The model under review builds one solid part; all positions refer to its coordinate system, in mm. Round coordinates to 2 decimals unless told otherwise and drop trailing zeros. Order: outer loops, then holes, each group sorted by start corner. A loop starts at its lowest first (then second) coordinate and runs counter-clockwise, first axis right, second up. Notation, with made-up numbers: M 27.25,27.25 L 83.25,27.25 A33 cw 83.25,61.25 Z; hole C -8.5,6.5 d8. An arc over 180 degrees is marked long. Answer as a JSON object with one key per item and string values. Group by question number.
1) Consider section A-A, the plane y = 1.5. Count the separate pieces of the cut face and the enclosed holes in it, then the cut area to 3 significant figures.
2) The part is to be moulded in two halves that separate along X. For faces 1 (the flat face through (69.85, 13, 11)), 2 (the flat face through (5, 3.175, -2)), 3 (the flat face through (-47.5, 1.6, -3.3)), 4 (the cylindrical face through (27.93, 1.57, -0.33)), say which applies: +X half, -X half, draft (parallel to the pull), parting line (faces both ways), or undercut.
3) Insertion check: pin 1 Ø8 at (x, z) = (-25.4, 0) entering from +Y (3 decimals); pin 2 Ø6 at (x, y) = (44.45, 17.46) entering from -Z (3 decimals); pin 3 Ø8 at (y, z) = (5.5, -2.5) entering from +X. Each pin has a flat end and moves straight along its axis. Give the tip position at first contact, or say it passes through.
4) Consider section D-D, the plane x = 19.05. Write out the cut boundary in (y, z) (3 decimals).
5) Consider section C-C, the plane z = 4.5. Write out the cut boundary in (x, y) (3 decimals), then the cut area to 3 significant figures.
6) To check wall thickness, follow line 1 (Y direction, x = -44.45, z = 10.7); line 2 (Y direction, x = 16.5, z = 0.5) (3 decimals); line 3 (Z direction, x = 42, y = 23) (3 decimals). State the ranges of each line that lie inside material, in increasing order.
7) Consider section B-B, the plane x = -44.45. Write out the cut boundary in (y, z) (3 decimals).
```python
from build123d import *

# Parameters (mm, degrees)
SKETCH2_W           = 127
SKETCH2_H           = 25.4
SKETCH2_R           = 2.5527
BOSS_EXTRUDE1_DEPTH = 3.175
SKETCH4_W           = 127
SKETCH4_H           = 22.225
SKETCH4_R           = 2.5527
BOSS_EXTRUDE3_DEPTH = 3.175
CUT_EXTRUDE1_DEPTH  = 75.392628163


with BuildPart() as part:
    # Sketch2 → Boss-Extrude1 (new body)
    with BuildSketch(Plane(origin=(0, 0, 0), x_dir=(1, 0, 0), z_dir=(0, 1, 0))):
        with Locations((6.35, 0)):
            Rectangle(SKETCH2_W, SKETCH2_H)
        with Locations(Location((0, 0, 0), (0, 0, 270))):
            Circle(SKETCH2_R, mode=Mode.SUBTRACT)
        with Locations(Location((12.7, 0, 0), (0, 0, 270))):
            Circle(SKETCH2_R, mode=Mode.SUBTRACT)
        with Locations(Location((25.4, 0, 0), (0, 0, 270))):
            Circle(SKETCH2_R, mode=Mode.SUBTRACT)
        with Locations(Location((38.1, 0, 0), (0, 0, 270))):
            Circle(SKETCH2_R, mode=Mode.SUBTRACT)
        with Locations(Location((-12.7, 0, 0), (0, 0, 270))):
            Circle(SKETCH2_R, mode=Mode.SUBTRACT)
        with Locations(Location((-25.4, 0, 0), (0, 0, 270))):
            Circle(SKETCH2_R, mode=Mode.SUBTRACT)
        with Locations(Location((-38.1, 0, 0), (0, 0, 270))):
            Circle(SKETCH2_R, mode=Mode.SUBTRACT)
        with Locations(Location((50.8, 0, 0), (0, 0, 270))):
            Circle(SKETCH2_R, mode=Mode.SUBTRACT)
    extrude(amount=BOSS_EXTRUDE1_DEPTH)

    # Sketch4 → Boss-Extrude3 (add)
    with BuildSketch(Plane.XY.offset(12.7)):
        with Locations((6.35, 14.2875)):
            Rectangle(SKETCH4_W, SKETCH4_H)
        with Locations((6.35, 17.4625)):
            Circle(SKETCH4_R, mode=Mode.SUBTRACT)
        with Locations((19.05, 17.4625)):
            Circle(SKETCH4_R, mode=Mode.SUBTRACT)
        with Locations((31.75, 17.4625)):
            Circle(SKETCH4_R, mode=Mode.SUBTRACT)
        with Locations((44.45, 17.4625)):
            Circle(SKETCH4_R, mode=Mode.SUBTRACT)
        with Locations((57.15, 17.4625)):
            Circle(SKETCH4_R, mode=Mode.SUBTRACT)
        with Locations(Location((-44.45, 17.4625, 0), (0, 0, 180))):
            Circle(SKETCH4_R, mode=Mode.SUBTRACT)
        with Locations(Location((-31.75, 17.4625, 0), (0, 0, 180))):
            Circle(SKETCH4_R, mode=Mode.SUBTRACT)
        with Locations(Location((-19.05, 17.4625, 0), (0, 0, 180))):
            Circle(SKETCH4_R, mode=Mode.SUBTRACT)
        with Locations(Location((-6.35, 17.4625, 0), (0, 0, 180))):
            Circle(SKETCH4_R, mode=Mode.SUBTRACT)
    extrude(amount=-BOSS_EXTRUDE3_DEPTH)

    # Sketch5 → Cut-Extrude1 (cut, through all)
    with BuildSketch(Plane(origin=(0, 3.175, 0), x_dir=(1, 0, 0), z_dir=(0, 1, 0))):
        Polygon((-38.1, 12.7), (-57.15, -6.35), (-57.15, 12.7), align=None)
        Polygon((50.8, 12.7), (69.85, -6.35), (69.85, 12.7), align=None)
    extrude(amount=-CUT_EXTRUDE1_DEPTH, mode=Mode.SUBTRACT)


solid = part.part
```
Results list:
{
 "1": {"separate pieces": "1", "enclosed holes": "8", "area": "2,700 mm^2"},
 "2": {"face 1": "+X half", "face 2": "draft", "face 3": "-X half", "face 4": "undercut"},
 "3": {"pin 1": "y = 3.175", "pin 2": "z = 9.525", "pin 3": "x = 64.25"},
 "4": {"outline": "M 0,-12.7 L 3.175,-12.7 L 3.175,9.525 L 14.91,9.525 L 14.91,12.7 L 0,12.7 Z; M 20.015,9.525 L 25.4,9.525 L 25.4,12.7 L 20.015,12.7 Z"},
 "5": {"outline": "M -55.3,0 L 68,0 L 68,3.175 L -55.3,3.175 Z", "area": "391 mm^2"},
 "6": {"line 1": "0 to 14.91, 20.02 to 25.4", "line 2": "0 to 3.175", "line 3": "9.525 to 12.7"},
 "7": {"outline": "M 0,-6.35 L 3.175,-6.35 L 3.175,9.525 L 14.91,9.525 L 14.91,12.7 L 0,12.7 Z; M 20.015,9.525 L 25.4,9.525 L 25.4,12.7 L 20.015,12.7 Z"}
}
